Can you work these out from the model? Positions are in its coordinate system, mm. Face numbers are marked on the shaded views. A direction names the side the tool comes from. Coordinates: 2 decimals unless noted, no trailing zeros. Loops run counter-clockwise (first coordinate to the right, second up) from the corner with the lowest first, then second, coordinate; pieces in that order, holes last.
```python
from build123d import *

# Parameters (mm, degrees)
F0_R        = 4.25
F1_DEPTH    = 2.5
F2_W        = 30.2444149011
F2_H        = 3.5
F3_DEPTH    = 19.918
F5_R        = 1.75
F6_DEPTH    = 3
F8_D        = 4.4958
F9_T1_DEPTH = 2.5
F9_T3_DEPTH = 3
F9_T5_DEPTH = 28.5
F10_SIZE    = 5


# Not quite as in the source:
# - a fillet or chamfer that OpenCascade refuses, or shapes differently, is made with other operations: its cross-section is extruded or revolved along the edge and cut away or added


with BuildPart() as f1:
    # F0 (on Top) → F1 (new body)
    with BuildSketch(Plane.XY):
        with BuildLine():
            Line((-30.2444149011, 7.25), (-45, 7.25))
            ThreePointArc((-45, 7.25), (-52.25, 0), (-45, -7.25))
            Line((-45, -7.25), (-30.2444149011, -7.25))
            Line((-30.2444149011, -7.25), (-30.2444149011, -16.4255911708))
            Line((-30.2444149011, -16.4255911708), (0, -16.4255911708))
            Line((0, -16.4255911708), (0, 19))
            Line((0, 19), (-30.2444149011, 19))
            Line((-30.2444149011, 19), (-30.2444149011, 7.25))
        make_face()
        with Locations((-45, 0)):
            Circle(F0_R, mode=Mode.SUBTRACT)
    extrude(amount=F1_DEPTH)

    # F2 (on face) → F3 (join)
    with BuildSketch(Plane.XY.offset(2.5)):
        with Locations((-15.1222074506, 17.25)):
            Rectangle(F2_W, F2_H)
    extrude(amount=F3_DEPTH)

    # F4: F1 across plane


with BuildPart() as f1_1:
    add(f1.part)
    add(f1.part.mirror(Plane.YZ))

    # F5 (on face) → F6 (join)
    with BuildSketch(Plane.XY.offset(22.418)):
        with BuildLine():
            ThreePointArc((4.1231056256, 19), (4.9602824786, 20.5300878706), (5.25, 22.25))
            ThreePointArc((5.25, 22.25), (-1.7199121294, 27.2102824786), (-4.1231056256, 19))
            Line((-4.1231056256, 19), (4.1231056256, 19))
        make_face()
        with Locations((0, 22.25)):
            Circle(F5_R, mode=Mode.SUBTRACT)
    extrude(amount=-F6_DEPTH)

    # F8 (through all)
    with Locations(Plane(origin=(0, 0, 0), x_dir=(1, 0, 0), z_dir=(0, 0, -1))):
        with Locations((-22, 12), (22, 12)):
            Hole(F8_D / 2)

    # F9: fillet of radius 5 on 6 edges, made by hand

    # F9_s2 → F9_t1 (join)
    with BuildSketch(Plane.XY):
        with BuildLine():
            ThreePointArc((30.2444149011, 12.25), (31.7088809952, 8.7144660941), (35.2444149011, 7.25))
            Line((35.2444149011, 7.25), (30.2444149011, 7.25))
            Line((30.2444149011, 7.25), (30.2444149011, 12.25))
        make_face()
        with BuildLine():
            ThreePointArc((-35.2444149011, 7.25), (-31.7088809952, 8.7144660941), (-30.2444149011, 12.25))
            Line((-30.2444149011, 12.25), (-30.2444149011, 7.25))
            Line((-30.2444149011, 7.25), (-35.2444149011, 7.25))
        make_face()
    extrude(amount=F9_T1_DEPTH)

    # F9_s4 → F9_t3 (join)
    with BuildSketch(Plane.XY.offset(19.418)):
        with BuildLine():
            ThreePointArc((10.0995049384, 19), (6.8799003573, 20.1745397216), (5.1729171636, 23.1463414634))
            ThreePointArc((5.1729171636, 23.1463414634), (5.0894053491, 20.9614142663), (4.1231056256, 19))
            Line((4.1231056256, 19), (10.0995049384, 19))
        make_face()
        with BuildLine():
            ThreePointArc((-10.0995049384, 19), (-6.8799003573, 20.1745397216), (-5.1729171636, 23.1463414634))
            ThreePointArc((-5.1729171636, 23.1463414634), (-5.0894053491, 20.9614142663), (-4.1231056256, 19))
            Line((-4.1231056256, 19), (-10.0995049384, 19))
        make_face()
    extrude(amount=F9_T3_DEPTH)

    # F9_s6 → F9_t5 (cut)
    with BuildSketch(Plane.XZ.offset(-31.5)):
        with BuildLine():
            ThreePointArc((-30.2444149011, 17.418), (-28.7799488071, 20.9535339059), (-25.2444149011, 22.418))
            Line((-25.2444149011, 22.418), (-30.2444149011, 22.418))
            Line((-30.2444149011, 22.418), (-30.2444149011, 17.418))
        make_face()
        with BuildLine():
            ThreePointArc((25.2444149011, 22.418), (28.7799488071, 20.9535339059), (30.2444149011, 17.418))
            Line((30.2444149011, 17.418), (30.2444149011, 22.418))
            Line((30.2444149011, 22.418), (25.2444149011, 22.418))
        make_face()
    extrude(amount=F9_T5_DEPTH, mode=Mode.SUBTRACT)

    # F10
    f10_edges = [f1_1.edges().sort_by_distance(p)[0] for p in [
        (0, 19, 0),
        (0, 15.5, 2.5),
    ]]
    chamfer(f10_edges, length=F10_SIZE)


solid = f1_1.part
```
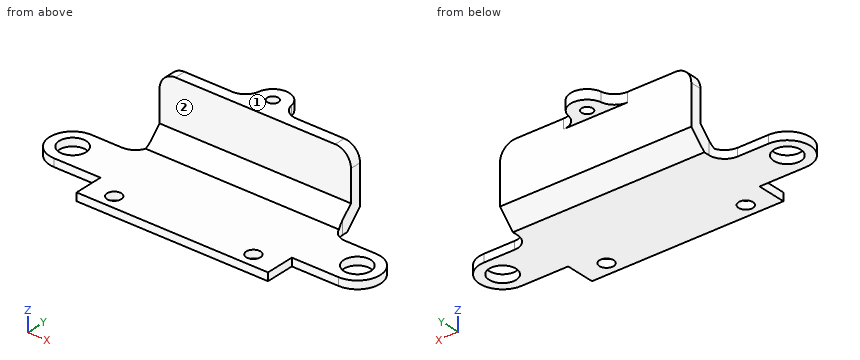
Item 1: Suppose I cut it at D-D, the plane z = 20.5. Please give me the cut outline in (x, y).
Results are:
outline: (-29.18, 15.5) - (29.18, 15.5) - (29.18, 19) - (10.1, 19) arc R5 cw to (5.17, 23.15) arc R5.25 ccw to (-5.17, 23.15) arc R5 cw to (-10.1, 19) - (-29.18, 19) - close; hole circle Ø3.5 at (0, 22.25)
Item 2: Suppose I cut it at B-B, the plane y = -12. Please give me the cut outline in (x, z), plus the area to 3 significant figures.
Results are:
outline: (-30.24, 0) - (-24.25, 0) - (-24.25, 2.5) - (-30.24, 2.5) - close; (-19.75, 0) - (19.75, 0) - (19.75, 2.5) - (-19.75, 2.5) - close; (24.25, 0) - (30.24, 0) - (30.24, 2.5) - (24.25, 2.5) - close
area: 129 mm2
Item 3: On a 3-axis mill with a long thin cutter (end or side, diameter ignored), from which of +Z, -Z, +X, -X, +Y, -Y can I reach the whole of each face in a straight line? I mean the marked faces 1 and 2. Say none if no direction works.
Results are:
face 1: +Z, +X, -X, +Y, -Y
face 2: +Z, +X, -X, -Y
Item 4: I'm going to push flat-ended pins straight in: P1, Ø10, axis at x = -8, y = -8, coming from the -Z side; P2, Ø7, axis at x = -45, y = 0, coming from the -Z side; P3, Ø3, axis at y = 17.5, z = 12, coming from the -X side; P4, Ø3, axis at x = -40, z = 1.5, coming from the +Y side. Where does each tip first touch, or does it pass through?
Results are:
P1: stops at z = 0
P2: passes through
P3: stops at x = -30.24
P4: stops at y = 7.25
Item 5: Suppose I cut it at A-A, the plane x = -22. Please give me the cut outline in (y, z), plus the area to 3 significant figures.
Results are:
outline: (-16.43, 0) - (-14.25, 0) - (-14.25, 2.5) - (-16.43, 2.5) - close; (-9.75, 0) - (14, 0) - (19, 5) - (19, 22.42) - (15.5, 22.42) - (15.5, 7.5) - (10.5, 2.5) - (-9.75, 2.5) - close
area: 147 mm2
Item 6: Suppose I cut it at C-C, the plane x = 14.5. Please give me the cut outline in (y, z), plus the area to 3 significant figures.
Results are:
outline: (-16.43, 0) - (14, 0) - (19, 5) - (19, 22.42) - (15.5, 22.42) - (15.5, 7.5) - (10.5, 2.5) - (-16.43, 2.5) - close
area: 158 mm2
Item 7: I need wall thicknesses on line 1 along X through (y, z) = (-12, 0.5); line 2 along Y through (x, z) = (-45, 1.65); line 3 along Y through (x, z) = (0, 21.1). Which ranges of each line are inside material? Lowest first, please.
Results are:
line 1: x = -30.24 to -24.25, -19.75 to 19.75, 24.25 to 30.24
line 2: y = -7.25 to -4.25, 4.25 to 7.25
line 3: y = 15.5 to 20.5, 24 to 27.5
